The model under review builds one solid part; all positions refer to its coordinate system, in mm. Face numbers are marked on the shaded views. A direction names the side the tool comes from. Round coordinates to 2 decimals unless told otherwise and drop trailing zeros. Loops run counter-clockwise (first coordinate to the right, second up) from the corner with the lowest first, then second, coordinate; pieces in that order, holes last. Notation, with made-up numbers: (54, 52.25) -> (81, 52.25) arc R16 ccw to (81, 77.25) -> close; hole circle Ø2 at (43.25, 68.5). An arc over 180 degrees is marked (long way). Return JSON: item names as keys, results as strings. Group by question number.
Autodesk Inventor part; units mm, degrees
ref_plane "YZ Plane" through (0, 0, 0) normal (1, 0, 0) x (0, 1, 0)
ref_plane "XZ Plane" through (0, 0, 0) normal (0, 1, 0) x (-1, 0, 0)
ref_plane "XY Plane" through (0, 0, 0) normal (0, 0, 1) x (1, 0, 0)
sketch "草图1" plane through (0, 0, 0) normal (0, 1, 0) x (-1, 0, 0)
  line L0 (0, 0) -> (-20, 0)
  line L1 (-20, 0) -> (-20, 25)
  line L2 (-20, 25) -> (0, 25)
  line L3 (0, 25) -> (0, 0)
  circle A0 centre (-5, 15.5) radius 1.65
  circle A1 centre (-5, 9.5) radius 1.6
  circle A2 centre (-5, 4) radius 1.55
  circle A3 centre (-5, 21) radius 1.7
  line L4 (0, 12.5) -> (-20, 12.5)
  line L5 (-10, 0) -> (-10, 25)
  circle A4 centre (-15, 15.5) radius 1.65
  circle A5 centre (-15, 9.5) radius 1.6
  circle A6 centre (-15, 4) radius 1.55
  circle A7 centre (-15, 21) radius 1.7
  line L6 (-11, 3) -> (-9, 3)
  line L7 (-9, 3) -> (-9, 18)
  line L8 (-9, 18) -> (-11, 18)
  line L9 (-11, 18) -> (-11, 3)
  line L10 (-11, 18) -> (-10, 21)
  line L11 (-9, 18) -> (-10, 21)
  dimension "d0" = 20
  dimension "d1" = 25
  dimension "d2" = 3.3
  dimension "d3" = 3.2
  dimension "d4" = 3.1
  dimension "d5" = 3.4
  dimension "d6" = 4
  dimension "d7" = 5
  dimension "d9" = 3
  dimension "d10" = 5
  dimension "d11" = 5
  dimension "d12" = 3
  dimension "d13" = 5
  dimension "d14" = 4
  dimension "d17" = 2
  dimension "d18" = 15
  dimension "d19" = 9
  dimension "d20" = 3
  dimension "d21" = 3
extrude "拉伸1" add sketch "草图1" along normal blind 5 contours L0 L5 L6 L7 L4 L3 | L0 L1 L4 L9 L6 L5 | L4 L7 L11 L5 L2 L3 | L1 L2 L5 L10 L9 L4
properties part number "PAACF测试板"
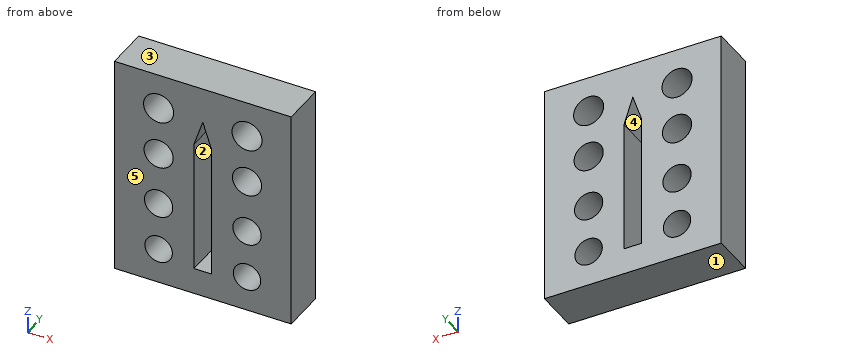
1. We need section A-A, the plane z = 13. Write out the cut boundary in (x, y), then the cut area to 3 significant figures.
2. Wall thickness on line 1 (Z direction, x = 15, y = 4.5); line 2 (X direction, y = 3.65, z = 7.75); line 3 (X direction, y = 1.2, z = 8.75): over which ranges is each line inside the solid? List them lowest first.
3. We need section B-B, the plane z = 4. Write out the cut boundary in (x, y).
4. Draft analysis for pull direction Z (two halves, no side actions). For the marked faces 1, 2 and 3, state which applies: pulls with the +Z half, pulls with the -Z half, needs draft (parallel to the pull), parting line crosses it, or undercut.
5. For P1, Ø4, axis at x = 15, z = 15.5, coming from the -Y side; P2, Ø2, axis at x = 5, z = 15.5, coming from the +Y side, all flat-tipped, find the tip position at first contact; note any pin that passes through.
6. We need section C-C, the plane y = 2.85. Give the number of separate pieces and of enclosed holes in the cut face, then the cut area to 3 significant figures.
7. We need section D-D, the plane x = 5. Write out the cut boundary in (y, z), then the cut area to 3 significant figures.
8. Tool access review of the marked faces 4 and 5: name each direction out of +Z, -Z, +X, -X, +Y, -Y from which nothing blocks a thin tool from reaching the whole face with its end or side.
Check sheet entries:
{
 "1": {"outline": "(0, 0) -> (9, 0) -> (9, 5) -> (0, 5) -> close; (11, 0) -> (20, 0) -> (20, 5) -> (11, 5) -> close", "area": "90.0 mm²"},
 "2": {"line 1": "z = 0 to 2.45, 5.55 to 7.9, 11.1 to 13.85, 17.15 to 19.3, 22.7 to 25", "line 2": "x = 0 to 9, 11 to 20", "line 3": "x = 0 to 3.59, 6.41 to 9, 11 to 13.59, 16.41 to 20"},
 "3": {"outline": "(0, 0) -> (3.45, 0) -> (3.45, 5) -> (0, 5) -> close; (6.55, 0) -> (9, 0) -> (9, 5) -> (6.55, 5) -> close; (11, 0) -> (13.45, 0) -> (13.45, 5) -> (11, 5) -> close; (16.55, 0) -> (20, 0) -> (20, 5) -> (16.55, 5) -> close"},
 "4": {"face 1": "pulls with the -Z half", "face 2": "undercut", "face 3": "pulls with the +Z half"},
 "5": {"P1": "stops at y = 0", "P2": "passes through"},
 "6": {"separate pieces": "1", "enclosed holes": "9", "area": "401 mm²"},
 "7": {"outline": "(0, 0) -> (5, 0) -> (5, 2.45) -> (0, 2.45) -> close; (0, 5.55) -> (5, 5.55) -> (5, 7.9) -> (0, 7.9) -> close; (0, 11.1) -> (5, 11.1) -> (5, 13.85) -> (0, 13.85) -> close; (0, 17.15) -> (5, 17.15) -> (5, 19.3) -> (0, 19.3) -> close; (0, 22.7) -> (5, 22.7) -> (5, 25) -> (0, 25) -> close", "area": "60.0 mm²"},
 "8": {"face 4": "+Y, -Y", "face 5": "+Z, -Z, +X, -X, -Y"}
}
